```python
from build123d import *

# Parameters (mm, degrees)
SKETCH1_R           = 2.25
SKETCH1_R_2         = 16.25
SKETCH1_R_3         = 4.25
SKETCH1_R_4         = 1.75
SKETCH1_R_5         = 9.75
BOSS_EXTRUDE1_DEPTH = 3
SKETCH2_R           = 1.25
CUT_EXTRUDE1_DEPTH  = 190.515777006


with BuildPart() as part:
    # Sketch1 → Boss-Extrude1 (new body)
    with BuildSketch(Plane.XY):
        with BuildLine():
            ThreePointArc((-137.970351553, -33.480224156), (-126.431132561, -39.888203569), (-124.422839539, -52.93360637))
            ThreePointArc((-124.422839539, -52.93360637), (-124.888175134, -64.31939994), (-119.594822483, -74.410646153))
            Line((-119.594822483, -74.410646153), (-92.540517723, -103.740413224))
            ThreePointArc((-92.540517723, -103.740413224), (-82.119700521, -108.557935129), (-71.344567605, -104.595807028))
            Line((-71.344567605, -104.595807028), (-37.221129556, -73.119733925))
            ThreePointArc((-37.221129556, -73.119733925), (-32.538343047, -69.892896145), (-27.140055215, -68.104192696))
            Line((-27.140055215, -68.104192696), (68.925058584, -50.795851294))
            ThreePointArc((68.925058584, -50.795851294), (82.107908339, -44.886103489), (91, -33.5))
            ThreePointArc((91, -33.5), (96.805715124, 7.17766304), (80.26119478, 44.789595257))
            ThreePointArc((80.26119478, 44.789595257), (69.434281248, 53.01522195), (56.08825014, 55.616461034))
            Line((56.08825014, 55.616461034), (-113.612398701, 49.485657112))
            ThreePointArc((-113.612398701, 49.485657112), (-129.404310002, 41.953312576), (-134.705774542, 25.279526249))
            ThreePointArc((-134.705774542, 25.279526249), (-136.343375771, 16.802270376), (-142.382746132, 10.632050724))
            ThreePointArc((-142.382746132, 10.632050724), (-155.099864059, -8.058287742), (-147.542861296, -29.364285714))
            ThreePointArc((-147.542861296, -29.364285714), (-143.125485566, -32.280163581), (-137.970351553, -33.480224156))
        make_face()
        with Locations((-81.514845762, -93.570135067)):
            Circle(SKETCH1_R, mode=Mode.SUBTRACT)
        with Locations((-103.42383694, -59.494238188)):
            Circle(SKETCH1_R_2, mode=Mode.SUBTRACT)
        with Locations((-138.3, -22.75)):
            Circle(SKETCH1_R, mode=Mode.SUBTRACT)
        with Locations((-138.3, -5.25)):
            Circle(SKETCH1_R, mode=Mode.SUBTRACT)
        with Locations((-68.3, -21.5)):
            Circle(SKETCH1_R, mode=Mode.SUBTRACT)
        with Locations((-74.1, 1.7)):
            Circle(SKETCH1_R, mode=Mode.SUBTRACT)
        with Locations((-65.4, 20.2)):
            Circle(SKETCH1_R, mode=Mode.SUBTRACT)
        with Locations((18.5, -8.7)):
            Circle(SKETCH1_R, mode=Mode.SUBTRACT)
        with Locations((8.1, 8.2)):
            Circle(SKETCH1_R, mode=Mode.SUBTRACT)
        with Locations((75.9, -21.8)):
            Circle(SKETCH1_R, mode=Mode.SUBTRACT)
        with Locations((40.017782272, 0)):
            Circle(SKETCH1_R_3, mode=Mode.SUBTRACT)
        with Locations((78, -0.1)):
            Circle(SKETCH1_R, mode=Mode.SUBTRACT)
        with Locations((73, 22.4)):
            Circle(SKETCH1_R, mode=Mode.SUBTRACT)
        with Locations((-114.213840088, 40.424858245)):
            Circle(SKETCH1_R_4, mode=Mode.SUBTRACT)
        with Locations((-111.422396488, 14.575141755)):
            Circle(SKETCH1_R_4, mode=Mode.SUBTRACT)
        with Locations((-125.742976533, 26.1042782)):
            Circle(SKETCH1_R_4, mode=Mode.SUBTRACT)
        with Locations((-112.818118288, 27.5)):
            Circle(SKETCH1_R_5, mode=Mode.SUBTRACT)
        with Locations((-99.893260043, 28.8957218)):
            Circle(SKETCH1_R_4, mode=Mode.SUBTRACT)
    extrude(amount=BOSS_EXTRUDE1_DEPTH)

    # Sketch2 → Cut-Extrude1 (cut, through all)
    with BuildSketch(Plane.XY.offset(3)):
        with Locations((56.232664601, 51.619068826)):
            Circle(SKETCH2_R)
        with Locations((-5.72691462, 49.380644672)):
            Circle(SKETCH2_R)
        with Locations((-67.686493842, 47.142220518)):
            Circle(SKETCH2_R)
        with Locations((68.215786874, -46.859236804)):
            Circle(SKETCH2_R)
        with Locations((7.198262283, -57.852948313)):
            Circle(SKETCH2_R)
        with Locations((-151.125466228, -14)):
            Circle(SKETCH2_R)
        with Locations((-53.819262309, -68.846659822)):
            Circle(SKETCH2_R)
    extrude(amount=-CUT_EXTRUDE1_DEPTH, mode=Mode.SUBTRACT)


solid = part.part
```
Here's how the part is built. I have some questions about the finished solid (model axes, mm). Coordinates: 2 decimals unless noted, no trailing zeros. Loops run counter-clockwise (first coordinate to the right, second up) from the corner with the lowest first, then second, coordinate; pieces in that order, holes last. Notation, with made-up numbers: (29.25, -24) - (84.25, -24) arc R11 cw to (84.25, -19) - close; hole circle Ø3 at (51.5, 27.25). An arc over 180 degrees is marked (long way). Answer as CSV lines item,"result".
Q1. If we section it at A-A, the plane x = -105.5: Write out the boundary of the cut face in (y, z).
Response:
outline,"(-89.69, 0) - (-75.61, 0) - (-75.61, 3) - (-89.69, 3) - close; (-43.38, 0) - (21.06, 0) - (21.06, 3) - (-43.38, 3) - close; (33.94, 0) - (49.78, 0) - (49.78, 3) - (33.94, 3) - close"
Q2. We'd pull the mould along X, two halves only. Please class faces 1 (the face through (-122.56, 27.93, 1.48)), 2 (the face through (-82.28, -108.55, 1.48)), 3 (the face through (-155.056, -7.733, 1.479)): pulls with the +X half, pulls with the -X half, needs draft (parallel to the pull), parting line crosses it, or undercut.
Response:
face 1,"undercut"
face 2,"parting line crosses it"
face 3,"pulls with the -X half"
Q3. If we section it at D-D, the plane x = 28: Write out the boundary of the cut face in (y, z).
Response:
outline,"(-58.17, 0) - (54.6, 0) - (54.6, 3) - (-58.17, 3) - close"
Q4. For pin 1 (1.5 mm diameter, centred on x = -5.73, y = 49.38, fed in from +Z); pin 2 (1.5 mm diameter, centred on y = 17.5, z = 0.5, fed in from +X), each with a flat end and sliding along its axis, tell me the tip position at first contact or that it passes through.
Response:
pin 1,"through"
pin 2,"x = 94.85"
Q5. If I drill on L1, parallel to X at y = 30, z = 2.2; L2, parallel to Y at x = -114, z = 0.75; L3, parallel to Y at x = -117, z = 0.55, over which ranges is the centre line in solid material (lowest first)? Write a range as [from, to].
Response:
L1,"[-134.68, -122.24], [-103.39, -101.25], [-98.54, 89.84]"
L2,"[-80.48, -71.83], [-47.16, 17.82], [37.18, 38.69], [42.16, 49.47]"
L3,"[-77.22, -68.42], [-50.56, 18.69], [36.31, 49.1]"
Q6. If we section it at C-C, the plane x = -13.5: Write out the boundary of the cut face in (y, z), and give its area (3 significant figures).
Response:
outline,"(-65.65, 0) - (53.1, 0) - (53.1, 3) - (-65.65, 3) - close"
area,"356 mm2"
Q7. If we section it at B-B, the plane z = 2.4: Give the number of separate pieces and of enclosed holes in the cut face, and give its area (3 significant figures).
Response:
separate pieces,"1"
enclosed holes,"25"
area,"27,000 mm2"
